Here's the drawing with two shaded views (mm, measured from the low corner). I have some questions. A direction names the side the tool comes from. Coordinates: 2 decimals unless noted, no trailing zeros. Write each loop counter-clockwise with the first axis right and the second up, starting at its lowest first coordinate (ties: lowest second). Pieces come first, ordered by that corner, then holes.
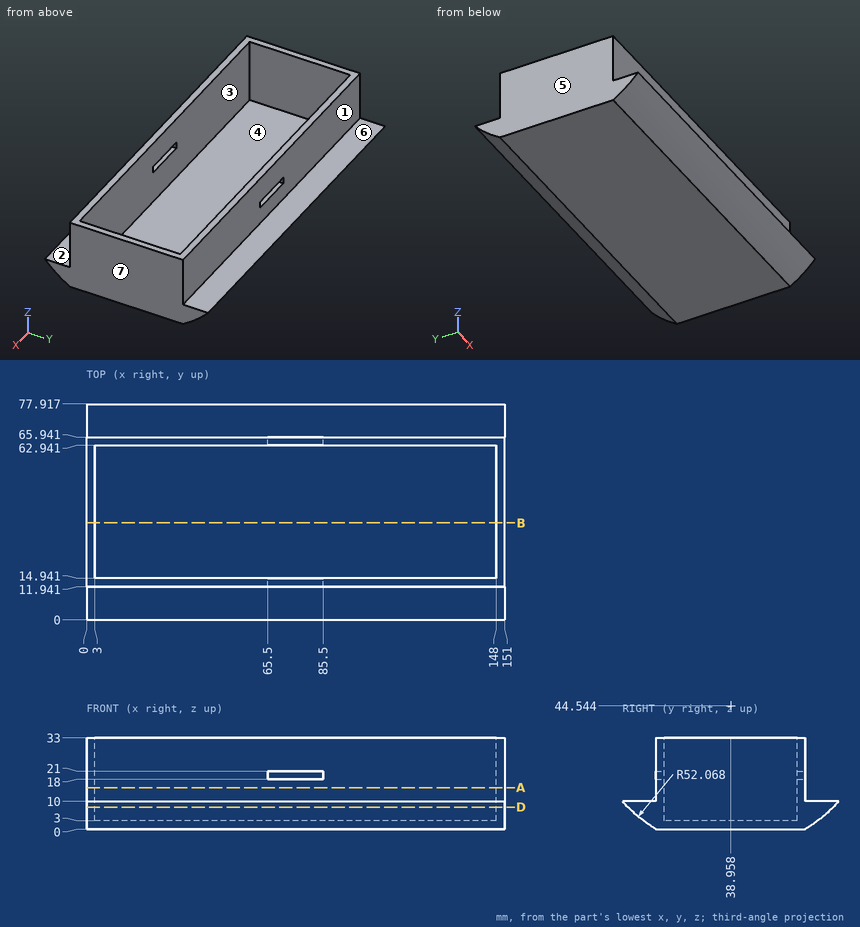
1. I want a section at D-D on z = 8. Please give me the cut outline in (x, y), plus the area to 3 significant figures.
Verdict:
outline: (0, 1.87) - (151, 1.87) - (151, 76.05) - (0, 76.05) - close; hole (3, 14.94) - (148, 14.94) - (148, 62.94) - (3, 62.94) - close
area: 4,240 mm2
2. I want a section at A-A on z = 15. Please give me the cut outline in (x, y), plus the area to 3 significant figures.
Verdict:
outline: (0, 11.94) - (151, 11.94) - (151, 65.94) - (0, 65.94) - close; hole (3, 14.94) - (148, 14.94) - (148, 62.94) - (3, 62.94) - close
area: 1,190 mm2
3. For pin 1 (1 mm diameter, centred on x = 33.5, y = 35.5, fed in from +Z); pin 2 (2 mm diameter, centred on x = 38.5, z = 23, fed in from +Y); pin 3 (3.5 mm diameter, centred on x = 57.5, y = 7.5, fed in from +Z), each with a flat end and sliding along its axis, tell me the tip position at first contact or that it passes through.
Verdict:
pin 1: stops at z = 3
pin 2: stops at y = 65.94
pin 3: stops at z = 10
4. On a 3-axis mill with a long thin cutter (end or side, diameter ignored), from which of +Z, -Z, +X, -X, +Y, -Y can I reach the whole of each face in a straight line? I mean the marked faces 1, 2 and 3. Say none if no direction works.
Verdict:
face 1: +Z, +X, -X, +Y
face 2: +Z, +X, -X, -Y
face 3: +Z
5. I want a section at B-B on y = 35. Please give me the cut outline in (x, z), plus the area to 3 significant figures.
Verdict:
outline: (0, 0) - (151, 0) - (151, 33) - (148, 33) - (148, 3) - (3, 3) - (3, 33) - (0, 33) - close
area: 633 mm2
6. If we mould it in two halves opening along X, with no side actions, what happens to the marked faces 4, 5, 6 and 7? For each: pulls with the +X half, pulls with the -X half, needs draft (parallel to the pull), parting line crosses it, or undercut.
Verdict:
face 4: undercut
face 5: pulls with the -X half
face 6: needs draft
face 7: pulls with the +X half
7. Please list where these lines run through material, in increasing order: line 1 along Y through (x, z) = (9, 12); line 2 along X through (y, z) = (44.5, 27); line 3 along Z through (x, y) = (102, 57.5).
Verdict:
line 1: y = 11.94 to 14.94, 62.94 to 65.94
line 2: x = 0 to 3, 148 to 151
line 3: z = 0 to 3
